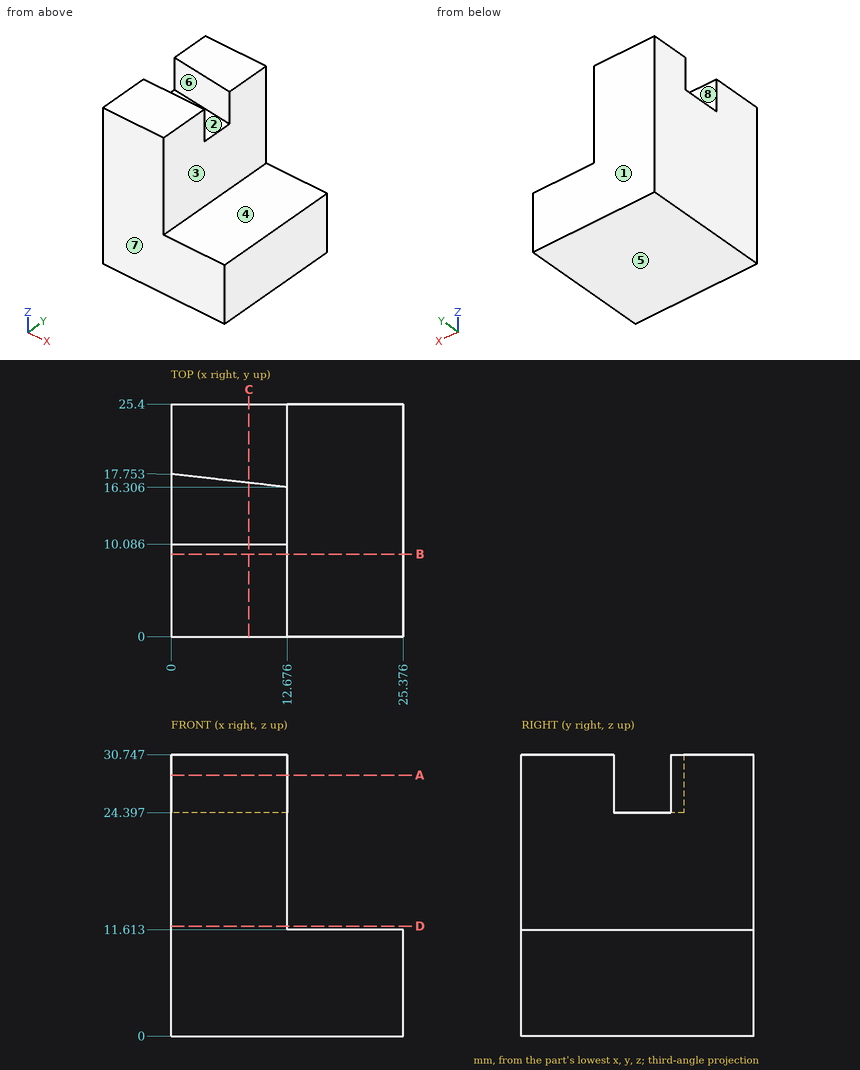
Design review of the part shown in the three views and the two pictorial views. Dimensions are in mm from the part's minimum x, y and z. A direction names the side the tool comes from. Give positions to 0.01 mm unless a question says otherwise; leave off trailing zeros. Write each loop counter-clockwise with the first axis right and the second up, starting at its lowest first coordinate (ties: lowest second). Pieces come first, ordered by that corner, then holes. Notation, with made-up numbers: (22, 57) -> (33, 57) arc R14 cw to (33, 75) -> close; hole circle Ø6 at (9, -7). An arc over 180 degrees is marked (long way). Answer in a Markdown table with one row per item.
1) Add section B-B on y = 9. State the section outline as (x, z) points (1 decimal), plus the area to 3 significant figures.
Worked answers:
| item | result |
|---|---|
| outline | (0, 0) -> (25.4, 0) -> (25.4, 11.6) -> (12.7, 11.6) -> (12.7, 30.7) -> (0, 30.7) -> close |
| area | 537 mm² |
2) Tool access review of the marked faces 4, 5, 6, 7 and 8: name each direction out of +Z, -Z, +X, -X, +Y, -Y from which nothing blocks a thin tool from reaching the whole face with its end or side.
Worked answers:
| item | result |
|---|---|
| face 4 | +Z, +X, +Y, -Y |
| face 5 | -Z, +X, -X, +Y, -Y |
| face 6 | +Z, -X |
| face 7 | +Z, -Z, +X, -X, -Y |
| face 8 | +Z, +X, -X |
3) Clearance check with flat-ended pins moving along their axes: P1, Ø6.5, axis at x = 19.5, y = 19, coming from the +Z side; P2, Ø6, axis at y = 16.5, z = 23.5, coming from the +X side. State where each tip first meets the part, or that it passes through.
Worked answers:
| item | result |
|---|---|
| P1 | z = 11.61 |
| P2 | x = 12.68 |
4) Mouldability with a two-part tool opening along Y and no side actions: class the marked faces 1, 2 and 3 as +Y half, -Y half, draft (parallel to the pull), parting line (faces both ways), or undercut.
Worked answers:
| item | result |
|---|---|
| face 1 | +Y half |
| face 2 | undercut |
| face 3 | draft |
5) Add section C-C on x = 8.5. State the section outline as (y, z) points.
Worked answers:
| item | result |
|---|---|
| outline | (0, 0) -> (25.4, 0) -> (25.4, 30.75) -> (16.78, 30.75) -> (16.78, 24.4) -> (10.09, 24.4) -> (10.09, 30.75) -> (0, 30.75) -> close |
6) Add section A-A on z = 28.5. State the section outline as (x, y) points (1 decimal).
Worked answers:
| item | result |
|---|---|
| outline | (0, 0) -> (12.7, 0) -> (12.7, 10.1) -> (0, 10.1) -> close; (0, 17.8) -> (12.7, 16.3) -> (12.7, 25.4) -> (0, 25.4) -> close |
7) Add section D-D on z = 12. State the section outline as (x, y) points (1 decimal), plus the area to 3 significant figures.
Worked answers:
| item | result |
|---|---|
| outline | (0, 0) -> (12.7, 0) -> (12.7, 25.4) -> (0, 25.4) -> close |
| area | 322 mm² |
8) For L1, parallel to X at y = 6.75, z = 24 (1 decimal); L2, parallel to Z at x = 12.75, y = 8.5; L3, parallel to Y at x = 10.75, z = 29 (1 decimal), list the stretches that pass through material, from the lowest coordinate up. Write a range as [from, to].
Worked answers:
| item | result |
|---|---|
| L1 | [0, 12.7] |
| L2 | [0, 11.61] |
| L3 | [0, 10.1], [16.5, 25.4] |
